The listing builds one solid part. Answer for the finished solid, in the listing's coordinates (mm). Coordinates: 2 decimals unless noted, no trailing zeros. Loops run counter-clockwise (first coordinate to the right, second up) from the corner with the lowest first, then second, coordinate; pieces in that order, holes last. Notation, with made-up numbers: M 20.5,-13 L 46.5,-13 A17 cw 46.5,12 Z; hole C 13,-11.75 d2. An arc over 180 degrees is marked long. Return JSON: item names as keys, results as strings. Group by question number.
1. Section A-A (y = -225.5) is taken. Write down the section's boundary in (x, z).
2. Section B-B (z = 0.55) is taken. Count the separate pieces of the cut face and the enclosed holes in it, then the cut area to 3 significant figures.
3. Given P1, Ø0.9, axis at y = 3, z = 2, coming from the +X side; P2, Ø1.5, axis at x = -8, z = 2, coming from the +Y side; P3, Ø0.9, axis at x = -7.5, z = 1.5, coming from the -Y side, each flat-ended and moving along its own axis, determine where each tip first touches the part or whether it passes through.
4. Straight lines are drawn through the part: L1, parallel to Y at x = -8.5, z = 0.5; L2, parallel to X at y = -82.5, z = 2.35. For each, find the intervals that lie inside material, in ascending order. Write a range as from..to.
```python
from build123d import *

# Parameters (mm, degrees)
F0_W     = 3
F0_H     = 36
F1_DEPTH = 3


with BuildPart() as f1:
    # F0 (on Top) → F1 (new body)
    with BuildSketch(Plane.XY):
        Polygon((-6.5, 5), (-6.5, 0), (-9.5, 0), (-9.5, 5), (-16, 5), (-16, 0), (-16, -270), (-16, -275), (-9.5, -275), (-9.5, -270), (-6.5, -270), (-6.5, -275), (0, -275), (0, -270), (0, 0), (0, 5), align=None)
        with Locations((-8, -237)):
            Rectangle(F0_W, F0_H, mode=Mode.SUBTRACT)
        with Locations((-8, -186)):
            Rectangle(F0_W, F0_H, mode=Mode.SUBTRACT)
        with Locations((-8, -135)):
            Rectangle(F0_W, F0_H, mode=Mode.SUBTRACT)
        with Locations((-8, -84)):
            Rectangle(F0_W, F0_H, mode=Mode.SUBTRACT)
        with Locations((-8, -33)):
            Rectangle(F0_W, F0_H, mode=Mode.SUBTRACT)
    extrude(amount=F1_DEPTH)


solid = f1.part
```
Worked out:
{
 "1": {"outline": "M -16,0 L -9.5,0 L -9.5,3 L -16,3 Z; M -6.5,0 L 0,0 L 0,3 L -6.5,3 Z"},
 "2": {"separate pieces": "1", "enclosed holes": "5", "area": "3,910 mm^2"},
 "3": {"P1": "x = 0", "P2": "y = 0", "P3": "y = -270"},
 "4": {"L1": "-270..-255, -219..-204, -168..-153, -117..-102, -66..-51, -15..0", "L2": "-16..-9.5, -6.5..0"}
}
